```python
from build123d import *

# Parameters (mm, degrees)
ESQUISSE1_R            = 2.35
FORME_PRINCIPALE_DEPTH = 10
ESQUISSE1_5_R          = 2.7
ECROU_DEPTH            = 6
ESQUISSE3_R            = 0.85
VIS_DEPTH              = 8


with BuildPart() as part:
    # Esquisse1 → forme principale (new body)
    with BuildSketch(Plane.XY):
        with BuildLine():
            Line((3, 9), (13, 11))
            ThreePointArc((13, 11), (18, 16), (13, 21))
            Line((13, 21), (3.169636963, 22.797308403))
            Line((3.169636963, 22.797308403), (-3.169636963, 22.797308403))
            Line((-3.169636963, 22.797308403), (-13, 21))
            ThreePointArc((-13, 21), (-18, 16), (-13, 11))
            Line((-13, 11), (-3, 9))
            Line((-3, 9), (-3, 6.5))
            Line((-3, 6.5), (-14.25, 6.5))
            Line((-14.25, 6.5), (-14.25, -6.5))
            Line((-14.25, -6.5), (14.25, -6.5))
            Line((14.25, -6.5), (14.25, 6.5))
            Line((14.25, 6.5), (3, 6.5))
            Line((3, 6.5), (3, 9))
        make_face()
        with Locations((-13, 16)):
            Circle(ESQUISSE1_R, mode=Mode.SUBTRACT)
        with Locations((13, 16)):
            Circle(ESQUISSE1_R, mode=Mode.SUBTRACT)
        Polygon((-2.396003617, 11.85), (2.396003617, 11.85), (4.792007234, 16), (2.396003617, 20.15), (-2.396003617, 20.15), (-4.792007234, 16), align=None, mode=Mode.SUBTRACT)
    extrude(amount=FORME_PRINCIPALE_DEPTH)

    # Esquisse1_5 → ecrou (add)
    with BuildSketch(Plane.XY):
        Polygon((-4.792007234, 16), (-2.396003617, 11.85), (2.396003617, 11.85), (4.792007234, 16), (2.396003617, 20.15), (-2.396003617, 20.15), align=None)
        with Locations((0, 16)):
            Circle(ESQUISSE1_5_R, mode=Mode.SUBTRACT)
    extrude(amount=ECROU_DEPTH)

    # Esquisse3 → vis (cut)
    with BuildSketch(Plane.XZ.offset(6.5)):
        with Locations((-9.25, 3)):
            Circle(ESQUISSE3_R)
        with Locations((0.45, 3)):
            Circle(ESQUISSE3_R)
    extrude(amount=-VIS_DEPTH, mode=Mode.SUBTRACT)


solid = part.part
```
Can you work these out from the model? Positions are in its coordinate system, mm. A direction names the side the tool comes from. Round coordinates to 2 decimals unless told otherwise and drop trailing zeros. Loops run counter-clockwise (first coordinate to the right, second up) from the corner with the lowest first, then second, coordinate; pieces in that order, holes last.
Item 1: Suppose I cut it at B-B, the plane y = -4.5. Write out the boundary of the cut face in (x, z), then the cut area to 3 significant figures.
Item 2: Suppose I cut it at C-C, the plane x = 0. Write out the boundary of the cut face in (y, z), then the cut area to 3 significant figures.
Item 3: Suppose I cut it at A-A, the plane z = 1. Write out the boundary of the cut face in (x, y), then the cut area to 4 significant figures.
Item 4: If we mould it in two halves opening along Y, with no side actions, what happens to faces 1 (the flat face through (0, 20.15, 8)), 2 (the flat face through (0, 22.797, 5)), 3 (the flat face through (-14.25, 0, 5))? For each: +Y half, -Y half, draft (parallel to the pull), parting line (faces both ways), or undercut.
Item 5: Please list where these lines run through material, in increasing order: L1, parallel to Y at x = -13, z = 7.25; L2, parallel to Z at x = -9.25, y = -3.75; L3, parallel to Y at x = -4, z = 9.
Item 6: Which directions (+Z, -Z, +X, -X, +Y, -Y) give clear straight access to the entire face, cutting with the end or side of a thin tool? Please do faces 4 (the flat face through (-9, 1.5, 3)), 5 (the flat face through (14.25, 0, 5)), 6 (the flat face through (3.61, 18.05, 7.97)), 7 (the flat face through (-3, 8, 5)).
Item 7: Suppose I cut it at D-D, the plane x = 13.5. Write out the boundary of the cut face in (y, z).
Item 8: Will these pins go through, and if not, where does the flat tip stop? pin 1 Ø3 at (y, z) = (7, 4) entering from -X; pin 2 Ø2.5 at (x, y) = (1.5, 16) entering from +Z; pin 3 Ø4 at (x, y) = (13, 16) entering from +Z; pin 4 Ø3 at (x, z) = (-6.5, 3) entering from +Y.
Reported:
1. outline: (-14.25, 0) - (14.25, 0) - (14.25, 10) - (-14.25, 10) - close; hole circle Ø1.7 at (-9.25, 3); hole circle Ø1.7 at (0.45, 3)
1. area: 280 mm2
2. outline: (-6.5, 0) - (13.3, 0) - (13.3, 6) - (11.85, 6) - (11.85, 10) - (-6.5, 10) - (-6.5, 3.72) - (1.5, 3.72) - (1.5, 2.28) - (-6.5, 2.28) - close; (18.7, 0) - (22.8, 0) - (22.8, 10) - (20.15, 10) - (20.15, 6) - (18.7, 6) - close
2. area: 216 mm2
3. outline: (-14.25, -6.5) - (14.25, -6.5) - (14.25, 6.5) - (3, 6.5) - (3, 9) - (13, 11) arc R5 ccw to (13, 21) - (3.17, 22.8) - (-3.17, 22.8) - (-13, 21) arc R5 ccw to (-13, 11) - (-3, 9) - (-3, 6.5) - (-14.25, 6.5) - close; hole circle Ø4.7 at (-13, 16); hole circle Ø5.4 at (0, 16); hole circle Ø4.7 at (13, 16)
3. area: 727.5 mm2
4. face 1: undercut
4. face 2: +Y half
4. face 3: draft
5. L1: y = -6.5 to 6.5, 11 to 13.65, 18.35 to 21
5. L2: z = 0 to 2.15, 3.85 to 10
5. L3: y = -6.5 to 6.5, 9.2 to 14.63, 17.37 to 22.65
6. face 4: -Y
6. face 5: +Z, -Z, +X, -Y
6. face 6: +Z
6. face 7: +Z, -Z, -X
7. outline: (-6.5, 0) - (6.5, 0) - (6.5, 10) - (-6.5, 10) - close; (11.03, 0) - (13.7, 0) - (13.7, 10) - (11.03, 10) - close; (18.3, 0) - (20.97, 0) - (20.97, 10) - (18.3, 10) - close
8. pin 1: stops at x = -14.25
8. pin 2: stops at z = 6
8. pin 3: passes through
8. pin 4: stops at y = 22.46
